For this review, take the finished solid that the model builds, in its own axes (mm). Coordinates: 2 decimals unless noted, no trailing zeros. Write each loop counter-clockwise with the first axis right and the second up, starting at its lowest first coordinate (ties: lowest second). Pieces come first, ordered by that corner, then holes.
1) We need section B-B on y = -76.2. Write out the cut boundary in (x, z).
2) Mouldability with a two-part tool opening along Y and no side actions: class faces 1 (the face through (-0.205, 142.877, 1.252)), 2 (the face through (-39.855, -147.096, 1.252)), 3 (the face through (-1.377, -100.745, 1.252)) as pulls with the +Y half, pulls with the -Y half, needs draft (parallel to the pull), parting line crosses it, or undercut.
3) We need section D-D on z = 2.15. Give the number of separate pieces and of enclosed holes in the cut face, then the cut area to 3 significant figures.
4) We need section A-A on x = 0. Write out the cut boundary in (y, z) (3 decimals).
5) We need section C-C on x = 38.1. Write out the cut boundary in (y, z).
6) Insertion check: P1, Ø1, axis at x = 48.5, z = 0.5, coming from the +Y side. The pin has a flat end and moves straight along its axis. Give the tip position at first contact, or say it passes through.
7) To check wall thickness, follow line 1 along Y through (x, z) = (0, 0.6) (3 decimals); line 2 along X through (y, z) = (52, 0.6); line 3 along Y through (x, z) = (4.5, 2.45). State the ranges of each line that lie inside material, in increasing order.
from build123d import *

# Parameters (mm, degrees)
SKETCH1_R           = 152.4
BOSS_EXTRUDE1_DEPTH = 2.54
SKETCH2_R           = 9.525
SKETCH2_R_2         = 6.35
CUT_EXTRUDE2_DEPTH  = 3.54
SKETCH4_R           = 6.35
CUT_EXTRUDE4_DEPTH  = 2.54


with BuildPart() as part:
    # Sketch1 → Boss-Extrude1 (new body)
    with BuildSketch(Plane.XY):
        Circle(SKETCH1_R)
    extrude(amount=BOSS_EXTRUDE1_DEPTH)

    # Sketch2 → Cut-Extrude2 (cut, through all)
    with BuildSketch(Plane.XY):
        with Locations((152.4, 0)):
            Circle(SKETCH2_R)
        with Locations((131.982271537, -76.2)):
            Circle(SKETCH2_R)
        with Locations((76.2, -131.982271537)):
            Circle(SKETCH2_R)
        with Locations((0, -152.4)):
            Circle(SKETCH2_R)
        with Locations((-76.2, -131.982271537)):
            Circle(SKETCH2_R)
        with Locations((-131.982271537, -76.2)):
            Circle(SKETCH2_R)
        with Locations((-152.4, 0)):
            Circle(SKETCH2_R)
        with Locations((-131.982271537, 76.2)):
            Circle(SKETCH2_R)
        with Locations((-76.2, 131.982271537)):
            Circle(SKETCH2_R)
        with Locations((0, 152.4)):
            Circle(SKETCH2_R)
        with Locations((76.2, 131.982271537)):
            Circle(SKETCH2_R)
        with Locations((131.982271537, 76.2)):
            Circle(SKETCH2_R)
        with Locations((38.1, 0)):
            Circle(SKETCH2_R_2)
        with Locations((0, -38.1)):
            Circle(SKETCH2_R_2)
        with Locations((-38.1, 0)):
            Circle(SKETCH2_R_2)
        with Locations((0, 38.1)):
            Circle(SKETCH2_R_2)
        with Locations((81.879271907, -47.273019677)):
            Circle(SKETCH2_R_2)
        with Locations((0, -94.546039353)):
            Circle(SKETCH2_R_2)
        with Locations((-81.879271907, -47.273019677)):
            Circle(SKETCH2_R_2)
        with Locations((-81.879271907, 47.273019677)):
            Circle(SKETCH2_R_2)
        with Locations((0, 94.546039353)):
            Circle(SKETCH2_R_2)
        with Locations((81.879271907, 47.273019677)):
            Circle(SKETCH2_R_2)
    extrude(amount=CUT_EXTRUDE2_DEPTH, mode=Mode.SUBTRACT)

    # Sketch4 → Cut-Extrude4 (cut)
    with BuildSketch(Plane.XY):
        Circle(SKETCH4_R)
    extrude(amount=CUT_EXTRUDE4_DEPTH, mode=Mode.SUBTRACT)


solid = part.part
Result:
1. outline: (-122.46, 0) - (122.46, 0) - (122.46, 2.54) - (-122.46, 2.54) - close
2. face 1: pulls with the +Y half
2. face 2: pulls with the -Y half
2. face 3: undercut
3. separate pieces: 1
3. enclosed holes: 11
3. area: 69,900 mm2
4. outline: (-142.875, 0) - (-100.896, 0) - (-100.896, 2.54) - (-142.875, 2.54) - close; (-88.196, 0) - (-44.45, 0) - (-44.45, 2.54) - (-88.196, 2.54) - close; (-31.75, 0) - (-6.35, 0) - (-6.35, 2.54) - (-31.75, 2.54) - close; (6.35, 0) - (31.75, 0) - (31.75, 2.54) - (6.35, 2.54) - close; (44.45, 0) - (88.196, 0) - (88.196, 2.54) - (44.45, 2.54) - close; (100.896, 0) - (142.875, 0) - (142.875, 2.54) - (100.896, 2.54) - close
5. outline: (-147.56, 0) - (-6.35, 0) - (-6.35, 2.54) - (-147.56, 2.54) - close; (6.35, 0) - (147.56, 0) - (147.56, 2.54) - (6.35, 2.54) - close
6. P1: stops at y = 144.64
7. line 1: y = -142.875 to -100.896, -88.196 to -44.45, -31.75 to -6.35, 6.35 to 31.75, 44.45 to 88.196, 100.896 to 142.875
7. line 2: x = -143.25 to -86.12, -77.64 to 77.64, 86.12 to 143.25
7. line 3: y = -144.01 to -99.03, -90.07 to -42.58, -33.62 to -4.48, 4.48 to 33.62, 42.58 to 90.07, 99.03 to 144.01
